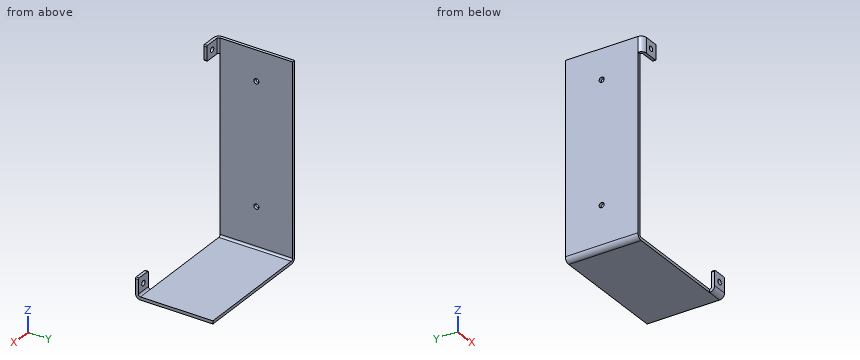
```python
from build123d import *

# Parameters (mm, degrees)
F1_DEPTH = 72
F3_DEPTH = 15
F5_DEPTH = 15
F6_R     = 1
F9_D     = 5
F11_D    = 5


with BuildPart() as f1:
    # F0 (on Front) → F1 (new body)
    with BuildSketch(Plane.XZ):
        with BuildLine():
            Line((0, 2), (0, 190))
            Line((0, 190), (-3, 190))
            Line((-3, 190), (-3, 2))
            ThreePointArc((-3, 2), (-1.535534, -1.535534), (2, -3))
            Line((2, -3), (120, -3))
            Line((120, -3), (120, 0))
            Line((120, 0), (2, 0))
            ThreePointArc((2, 0), (0.585786, 0.585786), (0, 2))
        make_face()
    extrude(amount=F1_DEPTH)

    # F2 (on face) → F3 (join)
    with BuildSketch(Plane.XY.offset(190)):
        with BuildLine():
            ThreePointArc((2, -74), (0.585786, -73.414214), (0, -72))
            Line((0, -72), (-3, -72))
            ThreePointArc((-3, -72), (-1.535534, -75.535534), (2, -77))
            Line((2, -77), (17, -77))
            Line((17, -77), (17, -74))
            Line((17, -74), (2, -74))
        make_face()
    extrude(amount=-F3_DEPTH)

    # F4 (on face) → F5 (join)
    with BuildSketch(Plane.YZ.offset(120)):
        with BuildLine():
            ThreePointArc((-72, 0), (-73.414214, 0.585786), (-74, 2))
            Line((-74, 2), (-74, 17))
            Line((-74, 17), (-77, 17))
            Line((-77, 17), (-77, 2))
            ThreePointArc((-77, 2), (-75.535534, -1.535534), (-72, -3))
            Line((-72, -3), (-72, 0))
        make_face()
    extrude(amount=-F5_DEPTH)

    # F6
    f6_edges = [f1.edges().sort_by_distance(p)[0] for p in [
        (120, -75.5, 17),
        (105, -75.5, 17),
        (17, -75.5, 190),
        (17, -75.5, 175),
    ]]
    fillet(f6_edges, radius=F6_R)

    # F9 (through all)
    with Locations(Plane.XZ.offset(77)):
        with Locations((9, 182.5), (112.5, 9)):
            Hole(F9_D / 2)

    # F11 (through all)
    with Locations(Plane(origin=(-3, 0, 0), x_dir=(0, -1, 0), z_dir=(-1, 0, 0))):
        with Locations((36, 160), (36, 40)):
            Hole(F11_D / 2)


solid = f1.part
```
Could you check a few things on this model? Use its own coordinates, in mm. Round coordinates to 2 decimals unless told otherwise and drop trailing zeros. Write each loop counter-clockwise with the first axis right and the second up, starting at its lowest first coordinate (ties: lowest second). Pieces come first, ordered by that corner, then holes. Notation, with made-up numbers: M -24,21.25 L 28,21.25 A27 cw 28,37.25 Z; hole C -29,-20 d5. An arc over 180 degrees is marked long. Answer in a Markdown table with one row per item. Add a question column.
Q1. Imagine slicing it at D-D (z = 9). Please give me the cut outline in (x, y).
Q2. Imagine slicing it at B-B (x = 9). Please give me the cut outline in (y, z).
Q3. Will these pins go through, and if not, where does the flat tip stop? pin 1 Ø1.5 at (x, y) = (110, -75) entering from +Z; pin 2 Ø4 at (x, z) = (9, 182.5) entering from +Y; pin 3 Ø2.5 at (y, z) = (-74, 6) entering from -X; pin 4 Ø1.5 at (y, z) = (-75, 185.5) entering from +X.
Q4. If I drill on line 1 (Y direction, x = -1.05, z = 160); line 2 (Z direction, x = 9, y = -75.8); line 3 (Z direction, x = -1.9, y = -36), over which ranges is the centre line in solid material (lowest first)? Write a range as from..to.
Q5. Imagine slicing it at A-A (z = 182.5). Please give me the cut outline in (x, y), then the cut area to 3 significant figures.
Q6. Imagine slicing it at C-C (y = -36). Please give me the cut outline in (x, z), then the cut area to 3 significant figures.
Values:
| question | item | result |
|---|---|---|
| 1 | outline | M -3,-72 L 0,-72 L 0,0 L -3,0 Z; M 105,-77 L 110,-77 L 110,-74 L 105,-74 Z; M 115,-77 L 120,-77 L 120,-74 L 115,-74 Z |
| 2 | outline | M -77,175 L -74,175 L -74,180 L -77,180 Z; M -77,185 L -74,185 L -74,190 L -77,190 Z; M -72,-3 L 0,-3 L 0,0 L -72,0 Z |
| 3 | pin 1 | z = 17 |
| 3 | pin 2 | through |
| 3 | pin 3 | x = 105 |
| 3 | pin 4 | x = 17 |
| 4 | line 1 | -72..-38.5, -33.5..0 |
| 4 | line 2 | 175..180, 185..190 |
| 4 | line 3 | -1.13..37.5, 42.5..157.5, 162.5..190 |
| 5 | outline | M -3,-72 A5 ccw 2,-77 L 6.5,-77 L 6.5,-74 L 2,-74 A2 cw 0,-72 L 0,0 L -3,0 Z; M 11.5,-77 L 17,-77 L 17,-74 L 11.5,-74 Z |
| 5 | area | 262 mm^2 |
| 6 | outline | M -3,2 A5 ccw 2,-3 L 120,-3 L 120,0 L 2,0 A2 cw 0,2 L 0,37.5 L -3,37.5 Z; M -3,42.5 L 0,42.5 L 0,157.5 L -3,157.5 Z; M -3,162.5 L 0,162.5 L 0,190 L -3,190 Z |
| 6 | area | 904 mm^2 |
